Autodesk Inventor part; units mm, degrees
ref_plane "YZ Plane" through (0, 0, 0) normal (1, 0, 0) x (0, 1, 0)
ref_plane "XZ Plane" through (0, 0, 0) normal (0, 1, 0) x (-1, 0, 0)
ref_plane "XY Plane" through (0, 0, 0) normal (0, 0, 1) x (1, 0, 0)
sketch "Sketch9" plane through (0, 0, 0) normal (0, 1, 0) x (-1, 0, 0)
  line L0 (0, 0) -> (19.05, 0)
  line L1 (19.05, 0) -> (19.05, -76.2)
  line L2 (19.05, -76.2) -> (0, -76.2)
  line L3 (0, -76.2) -> (0, 0)
  circle A0 centre (9.525, -38.1) radius 0.9922
  circle A1 centre (9.525, -12.7) radius 0.9922
  circle A2 centre (9.525, -63.5) radius 0.9922
  dimension "d41" = 76.2
  dimension "d42" = 19.05
  dimension "d43" = 1.9844
  dimension "d44" = 9.525
  dimension "d45" = 38.1
  dimension "d46" = 1.9844
  dimension "d47" = 1.9844
  dimension "d48" = 9.525
  dimension "d49" = 9.525
  dimension "d50" = 25.4
  dimension "d51" = 25.4
extrude "Extrusion7" add sketch "Sketch9" along normal blind 3.175
sketch "Sketch10" plane through (0, 3.175, 0) normal (0, 1, 0) x (1, 0, 0)
  line L0 (-19.05, 76.2) -> (-19.05, 0)
  line L1 (-19.05, 0) -> (-22.225, 0)
  line L2 (-22.225, 0) -> (-22.225, 76.2)
  line L3 (-22.225, 76.2) -> (-19.05, 76.2)
  line L4 (-19.05, 76.2) -> (-19.05, 0)
  point P0 (0, 0)
  dimension "d54" = 3.175
  dimension "d55" = 76.2
extrude "Extrusion8" add sketch "Sketch10" against normal blind 22.225
sketch "Sketch11" plane through (-19.05, 0, 0) normal (1, 0, 0) x (0, 0, -1)
  circle A0 centre (25.4, -9.525) radius 0.9922
  circle A1 centre (50.8, -9.525) radius 0.9922
  line L0 (76.2, -19.05) -> (0, -19.05)
  line L1 (0, 0) -> (0, -19.05)
  dimension "d58" = 1.9844
  dimension "d59" = 1.9844
  dimension "d60" = 9.525
  dimension "d61" = 9.525
  dimension "d62" = 25.4
  dimension "d63" = 25.4
extrude "Extrusion9" cut sketch "Sketch11" against normal blind 22.225
sketch "Sketch12" plane through (0, 0, 0) normal (0, 0, 1) x (1, 0, 0)
  line L0 (-19.05, 0) -> (-19.05, -19.05)
  line L1 (-19.05, 0) -> (-19.2296, 0.1796)
  line L2 (-19.05, 0) -> (0, 0)
  line L3 (-19.2296, 0.1796) -> (0, 0.1796)
  line L4 (0, 0.1796) -> (0, -19.05)
  line L5 (0, -19.05) -> (-19.2296, -19.05)
  line L6 (-19.2296, -19.05) -> (-19.2296, 0.1796)
  point P0 (0, 0)
  dimension "d68" = 0.254
  dimension "d69" = 135
extrude "Extrusion10" cut sketch "Sketch12" against normal blind 76.2
fillet "Fillet4" radius 0.635 5 edges at (-22.225, -9.525, -24.4078) (-22.225, -9.525, -49.8078) (-8.5328, 3.175, -63.5) (-8.5328, 3.175, -38.1) (-8.5328, 3.175, -12.7)
sketch "Sketch13" plane through (0, 3.175, -76.2) normal (0, 0, -1) x (-1, 0, 0)
  line L0 (22.225, 0) -> (0, 0)
  line L1 (0, 0) -> (-3.175, 0)
  line L2 (-3.175, 0) -> (-3.175, -6.35)
  line L3 (-3.175, -6.35) -> (0, -6.35)
  line L4 (0, -6.35) -> (0, 0)
  point P0 (0, -3.175)
  dimension "d73" = 3.175
  dimension "d74" = 6.35
extrude "Extrusion11" add sketch "Sketch13" against normal blind 76.2
fillet "Fillet5" radius 2.54 1 edges at (0, -3.175, -38.1)
properties part number "Block Bracket Mark Guide Tool"
The model under review builds one solid part; all positions refer to its coordinate system, in mm. A direction names the side the tool comes from. Coordinates: 2 decimals unless noted, no trailing zeros. Write each loop counter-clockwise with the first axis right and the second up, starting at its lowest first coordinate (ties: lowest second). Pieces come first, ordered by that corner, then holes.
1) Clearance check with flat-ended pins moving along their axes: pin 1 Ø1.2 at (x, z) = (-9.525, -38.1) entering from +Y; pin 2 Ø9.5 at (x, z) = (-9.5, -41.5) entering from -Y; pin 3 Ø2.5 at (y, z) = (-9.525, -25.4) entering from +X; pin 4 Ø0.5 at (x, z) = (3, -53) entering from -Y (3 decimals). State where each tip first meets the part, or that it passes through.
2) The part is to be moulded in two halves that separate along Z. For faces 3 (the face through (-13.23, 0.35, -76.2)), 4 (the face through (-9.396, 1.343, -13.684)), 5 (the face through (0.724, -2.411, -37.567)), say which applies: pulls with the +Z half, pulls with the -Z half, needs draft (parallel to the pull), parting line crosses it, or undercut.
3) We need section A-A on z = -38.1. State the section outline as (x, y) points (3 decimals).
4) We need section B-B on y = -1.5. State the section outline as (x, z) points (3 decimals), then the cut area to 3 significant figures.
5) To check wall thickness, follow probe 1 along X at (y, z) = (1.1, -38.1) (3 decimals); probe 2 along Y at (x, z) = (-19.95, -25.4) (3 decimals); probe 3 along X at (y, z) = (-8.75, -33) (3 decimals). State the ranges of each line that lie inside material, in increasing order.
6) We need section C-C on z = -55.5. State the section outline as (x, y) points (3 decimals), then the cut area to 3 significant figures.
7) Machinability: for faces 1 (the face through (-19.23, -10, -38)), 2 (the face through (-13, 3.175, -39)), which of the approach directions +Z, -Z, +X, -X, +Y, -Y give a long, thin tool a straight path to every point of the face, cutting with its end or side? Answer none if there is none.
Answer list:
1. pin 1: passes through
1. pin 2: stops at y = 0.18
1. pin 3: stops at x = -19.23
1. pin 4: stops at y = -3.175
2. face 3: pulls with the -Z half
2. face 4: undercut
2. face 5: needs draft
3. outline: (-22.225, -19.05) - (-19.23, -19.05) - (-19.23, 0.18) - (-10.517, 0.18) - (-10.517, 2.54) arc R0.635 ccw to (-11.152, 3.175) - (-22.225, 3.175) - close; (-8.533, 0.18) - (0, 0.18) - (0, -0.635) arc R2.54 ccw to (2.54, -3.175) - (3.175, -3.175) - (3.175, 3.175) - (-7.898, 3.175) arc R0.635 ccw to (-8.533, 2.54) - close
4. outline: (-22.225, -76.2) - (-19.23, -76.2) - (-19.23, 0) - (-22.225, 0) - close; (0.152, -76.2) - (3.175, -76.2) - (3.175, 0) - (0.152, 0) - close
4. area: 459 mm2
5. probe 1: x = -22.225 to -10.517, -8.533 to 3.175
5. probe 2: y = -19.05 to -10.517, -8.533 to 3.175
5. probe 3: x = -22.225 to -19.23
6. outline: (-22.225, -19.05) - (-19.23, -19.05) - (-19.23, 0.18) - (0, 0.18) - (0, -0.635) arc R2.54 ccw to (2.54, -3.175) - (3.175, -3.175) - (3.175, 3.175) - (-22.225, 3.175) - close
6. area: 143 mm2
7. face 1: +Z, -Z, -Y
7. face 2: +Z, -Z, +X, -X, +Y
